Verification items for this drawing (mm, ordinates from the low corner). A direction names the side the tool comes from. Give positions to 0.01 mm unless a question says otherwise; leave off trailing zeros. Loops run counter-clockwise (first coordinate to the right, second up) from the corner with the lowest first, then second, coordinate; pieces in that order, holes last. Notation, with made-up numbers: M 38,1.5 L 45,1.5 A17 ccw 45,7.5 Z; hole C -36.75,25.25 d2. An arc over 180 degrees is marked long. Put each result on its own line as item: value. Start each with the question number.
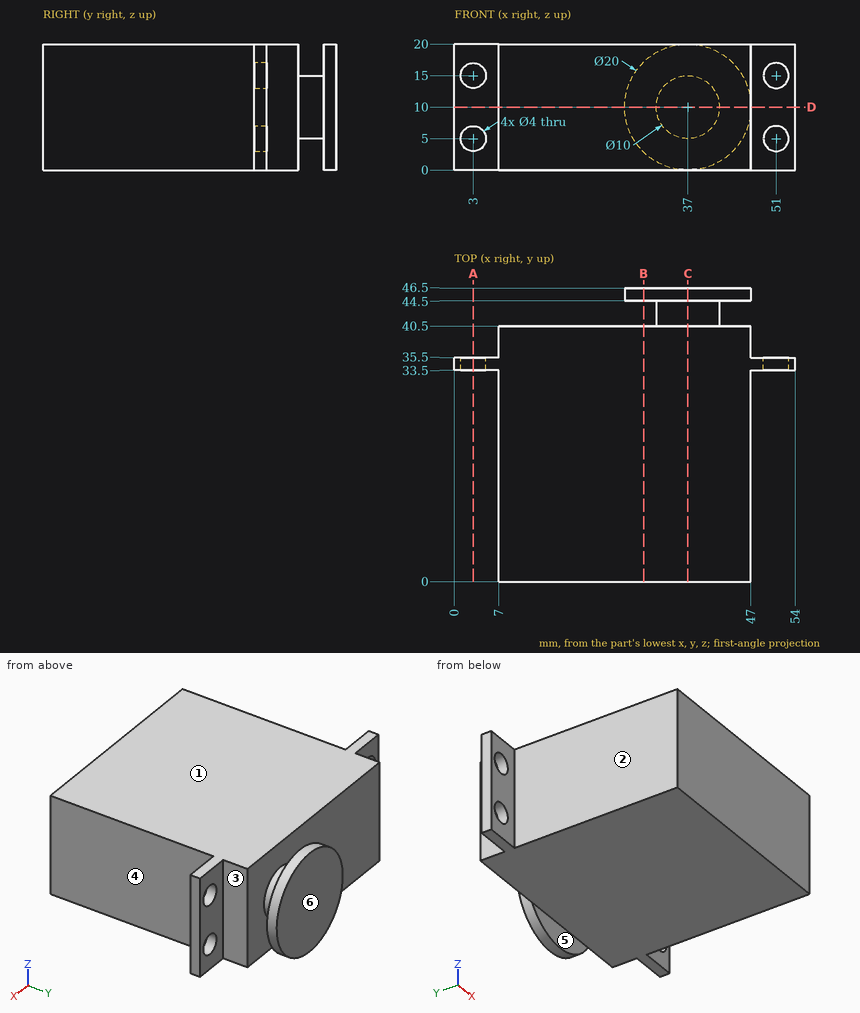
Q1. Go/stop test with flat-tipped pins: pin 1 (1 mm diameter, centred on y = 30.5, z = 4, fed in from +X); pin 2 (4 mm diameter, centred on x = 32.5, y = 22.5, fed in from -Z); pin 3 (1.5 mm diameter, centred on y = 27, z = 17.5, fed in from -X); pin 4 (7.5 mm diameter, centred on x = 51.5, z = 14, fed in from +Y). Record where each tip stops, or that it passes through.
Q2. Scan lines: L1, parallel to X at y = 34.5, z = 5; L2, parallel to Y at x = 42.5, z = 6.5; L3, parallel to Y at x = 19, z = 13.25. Record each from-to range of solid material in increasing order.
Q3. Cross-section at D-D, the plane z = 10. Record the boundary of the cut face in (x, y).
Q4. Cross-section at B-B, the plane x = 30. Record the boundary of the cut face in (y, z).
Q5. Release check for a two-part mould opening along Y. For the marked faces 4, 5 and 6 record: pulls with the +Y half, pulls with the -Y half, needs draft (parallel to the pull), parting line crosses it, or undercut.
Q6. Cross-section at C-C, the plane x = 37. Record the boundary of the cut face in (y, z), then the cut area to 3 significant figures.
Q7. Set-up check for the marked faces 1, 2 and 3: record each of +Z, -Z, +X, -X, +Y, -Y from which the full face is reachable in a straight line by a thin tool's end or side.
Q8. Cross-section at A-A, the plane x = 3. Record the boundary of the cut face in (y, z).
Ans:
1. pin 1: stops at x = 47
1. pin 2: stops at z = 0
1. pin 3: stops at x = 7
1. pin 4: stops at y = 35.5
2. L1: x = 0 to 1, 5 to 49, 53 to 54
2. L2: y = 0 to 40.5, 44.5 to 46.5
2. L3: y = 0 to 40.5
3. outline: M 0,33.5 L 7,33.5 L 7,0 L 47,0 L 47,33.5 L 54,33.5 L 54,35.5 L 47,35.5 L 47,40.5 L 42,40.5 L 42,44.5 L 47,44.5 L 47,46.5 L 27,46.5 L 27,44.5 L 32,44.5 L 32,40.5 L 7,40.5 L 7,35.5 L 0,35.5 Z
4. outline: M 0,0 L 40.5,0 L 40.5,20 L 0,20 Z; M 44.5,2.86 L 46.5,2.86 L 46.5,17.14 L 44.5,17.14 Z
5. face 4: needs draft
5. face 5: undercut
5. face 6: pulls with the +Y half
6. outline: M 0,0 L 40.5,0 L 40.5,5 L 44.5,5 L 44.5,0 L 46.5,0 L 46.5,20 L 44.5,20 L 44.5,15 L 40.5,15 L 40.5,20 L 0,20 Z
6. area: 890 mm^2
7. face 1: +Z, +X, -X, +Y, -Y
7. face 2: +Z, -Z, -X, -Y
7. face 3: +Z, -Z, +X, +Y
8. outline: M 33.5,0 L 35.5,0 L 35.5,3 L 33.5,3 Z; M 33.5,7 L 35.5,7 L 35.5,13 L 33.5,13 Z; M 33.5,17 L 35.5,17 L 35.5,20 L 33.5,20 Z
